Could you check a few things on this model? Use its own coordinates, in mm. A direction names the side the tool comes from. Round coordinates to 2 decimals unless told otherwise and drop trailing zeros. Answer as CSV lines item,"result". Start each with the question number.
Q1. Will these pins go through, and if not, where does the flat tip stop? pin 1 Ø4 at (x, y) = (-1, 40) entering from +Z; pin 2 Ø4 at (y, z) = (65.5, -184.5) entering from +X.
Q2. If I drill on line 1 (Y direction, x = 52, z = -184); line 2 (Y direction, x = 64.5, z = -187.5); line 3 (Z direction, x = 19, y = 10.5), over which ranges is the centre line in solid material (lowest first)? Write a range as [from, to].
Q3. If we mould it in two halves opening along Z, with no side actions, what happens to faces 3 (the cylindrical face through (64.08, 32.18, -183.35)), 4 (the flat face through (25, 48, -192.5)), 5 (the cylindrical face through (61.292, 91.526, -184.345)), 6 (the flat face through (41, 97, -187))? For each: pulls with the +Z half, pulls with the -Z half, needs draft (parallel to the pull), parting line crosses it, or undercut.
Q4. Imagine slicing it at A-A on y = 31. Give the number of separate pieces and of enclosed holes in the cut face, and give its area (3 significant figures).
Q5. For faces 1 (the flat face through (0, 48, -187.5)), 2 (the cylindrical face through (0, 29, -190)), which set-ups out of +Z, -Z, +X, -X, +Y, -Y let a thin tool reach every point of the face, with its end or its side?
from build123d import *

# Parameters (mm, degrees)
BOSS_EXTRUDE1_DEPTH = 120
SKETCH7_R           = 2
SKETCH7_W           = 65
SKETCH7_H           = 23
CUT_EXTRUDE3_DEPTH  = 20
SKETCH8_R           = 1.75
CUT_EXTRUDE4_DEPTH  = 20


with BuildPart() as part:
    # Sketch2 → Boss-Extrude1 (new body)
    with BuildSketch(Plane(origin=(0, 0, 0), x_dir=(1, 0, 0), z_dir=(0, 1, 0))):
        with BuildLine():
            Line((7.497222042, 192.5), (58, 192.5))
            Line((58, 192.5), (72.130758111, 187.482989601))
            Line((72.130758111, 187.482989601), (72.329757157, 187.411039321))
            Line((72.329757157, 187.411039321), (67.777738536, 174.8211319))
            add(Edge.make_bspline(
                [(58, 178.303813756), (62.937238269, 176.697757749), (67.777738536, 174.8211319)],
                knots=[0, 0, 0, 1, 1, 1], degree=2))
            add(Edge.make_bspline(
                [(6, 187.5), (32.674168427, 186.491531402), (58, 178.303813756)],
                knots=[0, 0, 0, 1, 1, 1], degree=2))
            Line((6, 187.5), (-7, 187.5))
            Line((-7, 187.5), (-7, 192.5))
            Line((-7, 192.5), (7.497222042, 192.5))
        make_face()
    extrude(amount=BOSS_EXTRUDE1_DEPTH)

    # Sketch7 → Cut-Extrude3 (cut)
    with BuildSketch(Plane(origin=(0, 0, -192.5), x_dir=(-1, 0, 0), z_dir=(0, 0, -1))):
        with Locations((-17, 6)):
            Circle(SKETCH7_R)
        with Locations((-52, 6)):
            Circle(SKETCH7_R)
        with Locations((-17, 91)):
            Circle(SKETCH7_R)
        with Locations((-52, 91)):
            Circle(SKETCH7_R)
        with Locations((0, 31)):
            Circle(SKETCH7_R)
        with Locations((0, 91)):
            Circle(SKETCH7_R)
        with Locations((-25.5, 108.5)):
            Rectangle(SKETCH7_W, SKETCH7_H)
    extrude(amount=-CUT_EXTRUDE3_DEPTH, mode=Mode.SUBTRACT)

    # Sketch8 → Cut-Extrude4 (cut)
    with BuildSketch(Plane(origin=(67.187435243, 0, -189.238076061), x_dir=(-0.9423674008829427, 0, -0.33457985855865147), z_dir=(0.33457985855865147, 0, -0.9423674008829428))):
        with Locations((2.249313521, 31)):
            Circle(SKETCH8_R)
        with Locations((2.249313521, 91)):
            Circle(SKETCH8_R)
        Polygon((9.749313521, 97), (-5.245642901, 97), (-14.139279105, 97), (-14.139279105, 120), (-5.245642901, 120), (9.749313521, 120), align=None)
    extrude(amount=-CUT_EXTRUDE4_DEPTH, mode=Mode.SUBTRACT)


solid = part.part
Checks:
1,pin 1,"z = -187.5"
1,pin 2,"x = 72"
2,line 1,"[0, 4], [8, 89], [93, 97]"
2,line 2,"[0, 29.28], [32.72, 89.28], [92.72, 97]"
2,line 3,"[-192.5, -186.57]"
3,face 3,"undercut"
3,face 4,"pulls with the -Z half"
3,face 5,"undercut"
3,face 6,"needs draft"
4,separate pieces,"3"
4,enclosed holes,"0"
4,area,"604 mm^2"
5,face 1,"+Z, -X, +Y, -Y"
5,face 2,"+Z, -Z"
